Check sheet for the modelled part. Datum: model origin and axes. Units: mm. Face numbers are marked on the shaded views. A direction names the side the tool comes from. Give positions to 0.01 mm unless a question says otherwise; leave off trailing zeros. Order: outer loops, then holes, each group sorted by start corner. A loop starts at its lowest first (then second) coordinate and runs counter-clockwise, first axis right, second up. Notation, with made-up numbers: (14.5, -21) -> (61.5, -21) arc R34 ccw to (61.5, 16) -> close; hole circle Ø10 at (-37, -25.75). An arc over 180 degrees is marked (long way). Answer in a Markdown table with one row per item. Add a question column.
(1) Go/stop test with flat-tipped pins: pin 1 (8 mm diameter, centred on x = 0.5, y = 6, fed in from +Z); pin 2 (6 mm diameter, centred on x = 7, z = 47, fed in from -Y); pin 3 (4.5 mm diameter, centred on x = 1.5, y = -6, fed in from -Z); pin 4 (0.8 mm diameter, centred on x = -5.5, z = 50, fed in from +Y). Record where each tip stops, or that it passes through.
(2) Cross-section at A-A (x = -7). Record the cut outline in (y, z).
(3) Set-up check for the marked faces 1, 2 and 3: record each of +Z, -Z, +X, -X, +Y, -Y from which the full face is reachable in a straight line by a thin tool's end or side.
(4) Cross-section at D-D (x = -15). Record the cut outline in (y, z).
(5) Release check for a two-part mould opening along X. For the marked faces 4, 5 and 6 record: released by +X, released by -X, zero draft, split by the parting line, or undercut.
(6) Cross-section at B-B (z = 42.5). Record the cut outline in (x, y), then the cut area to 3 significant figures.
(7) Cross-section at C-C (z = 53.75). Record the cut outline in (x, y).
(8) Thickness scan on L1, parallel to Y at x = 5, z = 52.5; L2, parallel to X at y = 12.75, z = 50.25; L3, parallel to Y at x = 7.5, z = 50.75. Record the ranges inside material, lowest first. Write a range as [from, to].
```python
from build123d import *

# Parameters (mm, degrees)
BOX068_W                  = 6
BOX068_H                  = 13
BOX068_DEPTH              = 55
CYLINDER051_R             = 6.35
CYLINDER051_DEPTH         = 55
BOX069_W                  = 6
BOX069_H                  = 13
BOX069_DEPTH              = 55
CYLINDER052_R             = 6.35
CYLINDER052_DEPTH         = 55
FUSION100_PLACEMENT_ANGLE = 180
CYLINDER050_R             = 7.35
CYLINDER050_DEPTH         = 55
CYLINDER_R                = 7.35
CYLINDER_DEPTH            = 60
BOX067_W                  = 62
BOX067_H                  = 55
BOX067_DEPTH              = 10
BOX066_W                  = 10
BOX066_H                  = 25
BOX066_DEPTH              = 20
BOX066_PLACEMENT_ANGLE    = 10
CYLINDER049_R             = 6.35
CYLINDER049_DEPTH         = 55
FUSION097_PLACEMENT_ANGLE = 180
BOX_W                     = 32
BOX_H                     = 25
BOX_DEPTH                 = 10
BOX065_W                  = 10
BOX065_H                  = 25
BOX065_DEPTH              = 20
BOX065_PLACEMENT_ANGLE    = 10
CYLINDER048_R             = 6.35
CYLINDER048_DEPTH         = 55


with BuildPart() as cube068:
    # Box068 → Box068 (new body)
    with BuildSketch(Plane(origin=(0, -6.5, 0), x_dir=(1, 0, 0), z_dir=(0, 0, 1))):
        with Locations((3, 6.5)):
            Rectangle(BOX068_W, BOX068_H)
    extrude(amount=BOX068_DEPTH)


with BuildPart() as fusion099:
    # Cylinder051 → Cylinder051 (new body)
    with BuildSketch(Plane(origin=(6, 0, 0), x_dir=(1, 0, 0), z_dir=(0, 0, 1))):
        Circle(CYLINDER051_R)
    extrude(amount=CYLINDER051_DEPTH)

    # Fusion099: union Cube068
    add(cube068.part)


with BuildPart() as cube069:
    # Box069 → Box069 (new body)
    with BuildSketch(Plane(origin=(0, -6.5, 0), x_dir=(1, 0, 0), z_dir=(0, 0, 1))):
        with Locations((3, 6.5)):
            Rectangle(BOX069_W, BOX069_H)
    extrude(amount=BOX069_DEPTH)


with BuildPart() as fusion101:
    # Cylinder052 → Cylinder052 (new body)
    with BuildSketch(Plane(origin=(6, 0, 0), x_dir=(1, 0, 0), z_dir=(0, 0, 1))):
        Circle(CYLINDER052_R)
    extrude(amount=CYLINDER052_DEPTH)

    # Fusion100: union Cube069
    add(cube069.part)


with BuildPart() as fusion101_1:
    # Fusion100 placement: moved
    add(fusion101.part.rotate(Axis((0, 0, 0), (0, 0, 1)), FUSION100_PLACEMENT_ANGLE))

    # Fusion101: union Fusion099
    add(fusion099.part)


with BuildPart() as obj1:
    # Cylinder050 → Cylinder050 (new body)
    with BuildSketch(Plane.XY):
        Circle(CYLINDER050_R)
    extrude(amount=CYLINDER050_DEPTH)


with BuildPart() as cylinder:
    # Cylinder → Cylinder (new body)
    with BuildSketch(Plane(origin=(15.5, 0, 0), x_dir=(1, 0, 0), z_dir=(0, 0, 1))):
        Circle(CYLINDER_R)
    extrude(amount=CYLINDER_DEPTH)


with BuildPart() as cube067:
    # Box067 → Box067 (new body)
    with BuildSketch(Plane(origin=(-27, -21.5, 55), x_dir=(1, 0, 0), z_dir=(0, 0, 1))):
        with Locations((31, 27.5)):
            Rectangle(BOX067_W, BOX067_H)
    extrude(amount=BOX067_DEPTH)


with BuildPart() as cube066:
    # Box066 → Box066 (new body)
    with BuildSketch(Plane.XY):
        with Locations((5, 12.5)):
            Rectangle(BOX066_W, BOX066_H)
    extrude(amount=BOX066_DEPTH)


with BuildPart() as cube066_1:
    # Box066 placement: moved
    add(cube066.part.moved(Location((11, -12.839144, 44.808394))).rotate(Axis((11, -12.839144, 44.808394), (-1, 0, 0)), BOX066_PLACEMENT_ANGLE))


with BuildPart() as fusion097:
    # Cylinder049 → Cylinder049 (new body)
    with BuildSketch(Plane.XY):
        Circle(CYLINDER049_R)
    extrude(amount=CYLINDER049_DEPTH)

    # Fusion097: union Cube066
    add(cube066_1.part)


with BuildPart() as fusion097_1:
    # Fusion097 placement: moved
    add(fusion097.part.rotate(Axis((0, 0, 0), (0, 0, 1)), FUSION097_PLACEMENT_ANGLE))


with BuildPart() as fusion:
    # Box → Box (new body)
    with BuildSketch(Plane(origin=(-16, -12.5, 45), x_dir=(1, 0, 0), z_dir=(0, 0, 1))):
        with Locations((16, 12.5)):
            Rectangle(BOX_W, BOX_H)
    extrude(amount=BOX_DEPTH)

    # Fusion: union Fusion097
    add(fusion097_1.part)


with BuildPart() as cube065:
    # Box065 → Box065 (new body)
    with BuildSketch(Plane.XY):
        with Locations((5, 12.5)):
            Rectangle(BOX065_W, BOX065_H)
    extrude(amount=BOX065_DEPTH)


with BuildPart() as cube065_1:
    # Box065 placement: moved
    add(cube065.part.moved(Location((11, -12.839144, 44.808394))).rotate(Axis((11, -12.839144, 44.808394), (-1, 0, 0)), BOX065_PLACEMENT_ANGLE))


with BuildPart() as cut003:
    # Cylinder048 → Cylinder048 (new body)
    with BuildSketch(Plane.XY):
        Circle(CYLINDER048_R)
    extrude(amount=CYLINDER048_DEPTH)

    # Fusion096: union Cube065
    add(cube065_1.part)

    # Fusion098: union Fusion
    add(fusion.part)

    # Cut: cut Cube067
    add(cube067.part, mode=Mode.SUBTRACT)

    # Cut001: cut Cylinder
    add(cylinder.part, mode=Mode.SUBTRACT)

    # Cut002: cut obj1
    add(obj1.part, mode=Mode.SUBTRACT)

    # Cut003: cut Fusion101
    add(fusion101_1.part, mode=Mode.SUBTRACT)


solid = cut003.part
```
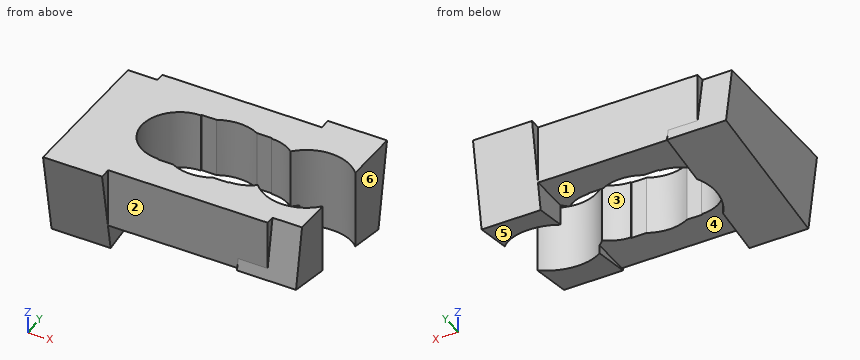
Answer below:
| question | item | result |
|---|---|---|
| 1 | pin 1 | stops at z = 55 |
| 1 | pin 2 | stops at y = -12.5 |
| 1 | pin 3 | stops at z = 45 |
| 1 | pin 4 | stops at y = 12.5 |
| 2 | outline | (-12.5, 45) -> (-6.27, 45) -> (-6.27, 55) -> (-12.5, 55) -> close; (6.27, 45) -> (12.5, 45) -> (12.5, 55) -> (6.27, 55) -> close |
| 3 | face 1 | -Z, +Y, -Y |
| 3 | face 2 | +Z, -Y |
| 3 | face 3 | +Z, -Z |
| 4 | outline | (-14.34, 55) -> (-11.78, 40.47) -> (12.84, 44.81) -> (12.5, 46.73) -> (12.5, 55) -> close |
| 5 | face 4 | undercut |
| 5 | face 5 | zero draft |
| 5 | face 6 | released by +X |
| 6 | outline | (-21, -12.14) -> (-11, -12.14) -> (-11, -3.91) arc R6.35 cw to (-12.34, -0.25) -> (-21, -0.25) -> close; (11, 5.81) arc R7.35 cw to (21, 4.88) -> (21, 12.14) -> (11, 12.14) -> close |
| 6 | area | 170 mm² |
| 7 | outline | (-21, -14.12) -> (-11, -14.12) -> (-11, -12.5) -> (16, -12.5) -> (16, -11.26) -> (21, -11.26) -> (21, -4.88) arc R7.35 cw to (10.03, -4.91) arc R6.35 cw to (6, -6.35) -> (6, -6.5) -> (3.43, -6.5) arc R7.35 cw to (-3.43, -6.5) -> (-6, -6.5) -> (-6, -6.35) arc R6.35 cw to (-6, 6.35) -> (-6, 6.5) -> (-3.43, 6.5) arc R7.35 cw to (3.43, 6.5) -> (6, 6.5) -> (6, 6.35) arc R6.35 cw to (10.03, 4.91) arc R7.35 cw to (21, 4.88) -> (21, 14.12) -> (11, 14.12) -> (11, 12.5) -> (-16, 12.5) -> (-16, 11.26) -> (-21, 11.26) -> close |
| 8 | L1 | y = [-12.5, -6.5], [6.5, 12.5] |
| 8 | L2 | x = [11, 21] |
| 8 | L3 | y = [-12.5, -6.17], [6.17, 12.5] |
